Input: part model. Units: mm. Frame: model coordinates. A direction names the side the tool comes from. Round coordinates to 2 decimals unless told otherwise and drop trailing zeros. Order: outer loops, then holes, each group sorted by start corner. A loop starts at its lowest first (then second) coordinate and runs counter-clockwise, first axis right, second up. Notation, with made-up numbers: (26.25, 14.25) -> (31.25, 14.25) arc R26 ccw to (31.25, 46.25) -> close; hole circle Ø8 at (-10, 24.25). An arc over 180 degrees is marked (long way). Use a Markdown table: item, result.
from build123d import *

# Parameters (mm, degrees)
CIRPATTERN1_COUNT   = 12
BOSS_EXTRUDE1_DEPTH = 4.445
BOSS_EXTRUDE2_DEPTH = 9.525
BOSS_EXTRUDE3_REACH = 69.945
SKETCH8_R           = 12.7


with BuildPart() as part:
    # Sketch1 → Revolve2 (revolve)
    with BuildSketch(Plane.XY):
        with BuildLine():
            add(Edge.make_bspline(
                [(0, 48.26), (-26.035, 48.26), (-26.035, 0)],
                knots=[3.141592654, 3.141592654, 3.141592654, 4.71238898, 4.71238898, 4.71238898], degree=2, weights=[1, 0.707106781, 1]))
            Line((-26.035, 0), (-15.875, 0))
            add(Edge.make_bspline(
                [(0, 38.1), (-15.875, 38.1), (-15.875, 0)],
                knots=[3.141592654, 3.141592654, 3.141592654, 4.71238898, 4.71238898, 4.71238898], degree=2, weights=[1, 0.707106781, 1]))
            Line((0, 38.1), (0, 48.26))
        make_face()
    revolve(axis=Axis((-26.035, 0, 0), (1, 0, 0)))

    # Sketch2 → Cut-Loft1 section 0
    with BuildSketch(Plane(origin=(0, -34.29, 0), x_dir=(1, 0, 0), z_dir=(0, 1, 0)), mode=Mode.PRIVATE) as cut_loft1_s0:
        Polygon((0, 7.69896584), (-6.6675, -3.84948292), (6.6675, -3.84948292), align=None)
    cut_loft1 = loft([cut_loft1_s0.sketch, Vertex(0, -45.212, 0)], mode=Mode.SUBTRACT)

    # CirPattern1: Cut-Loft1 ×12 about axis
    cirpattern1_axis = Axis((0, 0, 0), (1, 0, 0))
    for i in range(1, CIRPATTERN1_COUNT):
        add(cut_loft1.rotate(cirpattern1_axis, i * 360 / CIRPATTERN1_COUNT), mode=Mode.SUBTRACT)

    # Sketch6 → Boss-Extrude1 (add)
    with BuildSketch(Plane(origin=(0, 0, 0), x_dir=(0, 0, -1), z_dir=(1, 0, 0))):
        Polygon((4.851243253, 42.407942289), (14.134652823, 40.27629228), (14.475716824, 41.761637811), (5.192307254, 43.89328782), align=None)
    boss_extrude1 = extrude(amount=BOSS_EXTRUDE1_DEPTH)

    # Sketch7 → Boss-Extrude2 (add)
    with BuildSketch(Plane(origin=(0, 1.065825004, 4.641704785), x_dir=(1, 0, 0), z_dir=(0, 0.223795276, 0.974636175))):
        Polygon((3.175, 42.418), (3.175, 41.148), (4.445, 42.418), align=None)
    boss_extrude2 = extrude(amount=-BOSS_EXTRUDE2_DEPTH)

    # Mirror1: Boss-Extrude1, Boss-Extrude2 across plane
    add(boss_extrude1.mirror(Plane(origin=(0, 0, 0), x_dir=(0, 0.223795276, 0.974636175), z_dir=(0, -0.974636175, 0.223795276))))
    add(boss_extrude2.mirror(Plane(origin=(0, 0, 0), x_dir=(0, 0.223795276, 0.974636175), z_dir=(0, -0.974636175, 0.223795276))))

    # Sketch8 → Boss-Extrude3 (add, up to next)
    with BuildSketch(Plane(origin=(-63.5, 0, 0), x_dir=(0, 0, -1), z_dir=(1, 0, 0)), mode=Mode.PRIVATE) as boss_extrude3_sk1:
        Circle(SKETCH8_R)
    boss_extrude3_tool1 = extrude(boss_extrude3_sk1.sketch, amount=BOSS_EXTRUDE3_REACH, mode=Mode.PRIVATE) - part.part
    add(boss_extrude3_tool1.solids().sort_by_distance((-63.5, 0, 0))[0])


solid = part.part
1) Pin query (flat end, axial travel): pin 1 Ø1.5 at (x, y) = (-10.5, -32.5) entering from +Z; pin 2 Ø6 at (x, y) = (-47, -16) entering from -Z; pin 3 Ø1 at (y, z) = (-41, 9.5) entering from -X; pin 4 Ø1.7 at (y, z) = (40, -10) entering from -X. Return the tip coordinate at first contact, or that it passes through.
Results found:
| item | result |
|---|---|
| pin 1 | stops at z = 31.07 |
| pin 2 | passes through |
| pin 3 | stops at x = -13.21 |
| pin 4 | stops at x = -14.26 |
2) Cut plane A-A on x = -54.5. Return loops of the section in (y, z), and give its area (3 significant figures).
Results found:
| item | result |
|---|---|
| outline | circle Ø25.4 at (0, 0) |
| area | 507 mm² |
3) Set-up query: faces 4 (the flat face through (4.445, -42, 10)), 5 (the flat face through (3.175, -41, 9)), 6 (the flat face through (3.175, 41, -9)). Return all of +Z, -Z, +X, -X, +Y, -Y with unobstructed straight access to the full face (end or side cutting, diameter ignored); none if empty.
Results found:
| item | result |
|---|---|
| face 4 | +Z, -Z, +X, +Y, -Y |
| face 5 | -Z, +Y |
| face 6 | +Z, -Y |
4) Line query: L1, parallel to Z at x = -2, y = -29; L2, parallel to X at y = -14.5, z = 38; L3, parallel to X at y = 4, z = 29.5. Output: solid intervals per line, ascending. Write a range as [from, to].
Results found:
| item | result |
|---|---|
| L1 | z = [-38.4, -24.24], [24.24, 38.4] |
| L2 | x = [-14.01, 0] |
| L3 | x = [-20.49, -9.91] |
5) Pull-direction query (Y, two-part tool) for faces 1 (the flat face through (4.445, 42, -10)), 2 (the flat face through (-2.011, -19.286, -34.482)), 3 (the flat face through (4, 41, -9)); classes: +Y half, -Y half, draft (parallel to the pull), parting line (faces both ways), or undercut.
Results found:
| item | result |
|---|---|
| face 1 | draft |
| face 2 | undercut |
| face 3 | -Y half |
